Input: part model. Units: mm. Frame: model coordinates. A direction names the side the tool comes from. Round coordinates to 2 decimals unless told otherwise and drop trailing zeros. Loops run counter-clockwise (first coordinate to the right, second up) from the corner with the lowest first, then second, coordinate; pieces in that order, holes last. Notation, with made-up numbers: (30, 0) -> (77, 0) arc R7 cw to (77, 11) -> close; hole circle Ø7 at (55, 5). An arc over 180 degrees is marked (long way). One line per question, with ' | ' between items. Start each with the question number.
Q1. Access query for faces 1 (the face through (-47, -47, 0)), 2 (the face through (47, -47, 0.414)), 3 (the face through (-14.33, 109.11, 1.2)). Directions: +Z, -Z, +X, -X, +Y, -Y. A direction counts if a zero-diameter tool reaches every point of the face in a straight line with its end or side. Return the directions, or none.
Q2. Material intervals for L1, parallel to Y at x = 0, z = 1.15; L2, parallel to Z at x = 50, y = -100; L3, parallel to X at y = 99.5, z = 1.2, sorted ascending.
Q3. Contact query for a flat-ended pin moving along its axis: P1, Ø5, axis at x = 75.5, y = 37.5, coming from the +Z side. Output: stop coordinate, or through.
Q4. Cut plane A-A on y = 0. Return loops of the section in (x, z), and give its area (3 significant figures).
from build123d import *

# Parameters (mm, degrees)
F2_R     = 59.33948
F3_DEPTH = 25.4


with BuildPart() as f1:
    # F0 (on Front) → F1 (revolve)
    with BuildSketch(Plane.XZ):
        with BuildLine():
            Line((0, 0.414), (0, 0))
            Line((0, 0), (109.538073, 0))
            ThreePointArc((109.538073, 0), (109.89867, 0.149364), (110.048034, 0.509961))
            Line((110.048034, 0.509961), (110.048034, 1.878083))
            ThreePointArc((110.048034, 1.878083), (110.08374, 1.964284), (110.16994, 1.999989))
            Line((110.16994, 1.999989), (110.827769, 1.999989))
            Line((110.827769, 1.999989), (115.048034, 1.999989))
            Line((115.048034, 1.999989), (115.048034, 2.413989))
            Line((115.048034, 2.413989), (110.169929, 2.413989))
            ThreePointArc((110.169929, 2.413989), (109.790994, 2.257029), (109.634034, 1.878094))
            Line((109.634034, 1.878094), (109.634034, 0.509955))
            ThreePointArc((109.634034, 0.509955), (109.60593, 0.442105), (109.538079, 0.414))
            Line((109.538079, 0.414), (0, 0.414))
        make_face()
    revolve(axis=Axis((0, 0, 0.207), (0, 0, 1)))

    # F2 (on face) → F3 (cut)
    with BuildSketch(Plane.XY.offset(0.414)):
        Circle(F2_R)
    extrude(amount=-F3_DEPTH, mode=Mode.SUBTRACT)


solid = f1.part
Results:
1) face 1: -Z, +X, -X, +Y, -Y | face 2: +Z | face 3: -Z
2) L1: -110.05 to -109.63, 109.63 to 110.05 | L2: 2 to 2.41 | L3: -47.01 to -46.04, 46.04 to 47.01
3) P1: z = 0.41
4) outline: (-115.05, 2) -> (-110.17, 2) arc R0.12 cw to (-110.05, 1.88) -> (-110.05, 0.51) arc R0.51 ccw to (-109.54, 0) -> (-59.34, 0) -> (-59.34, 0.41) -> (-109.54, 0.41) arc R0.1 cw to (-109.63, 0.51) -> (-109.63, 1.88) arc R0.54 ccw to (-110.17, 2.41) -> (-115.05, 2.41) -> close; (59.34, 0) -> (109.54, 0) arc R0.51 ccw to (110.05, 0.51) -> (110.05, 1.88) arc R0.12 cw to (110.17, 2) -> (115.05, 2) -> (115.05, 2.41) -> (110.17, 2.41) arc R0.54 ccw to (109.63, 1.88) -> (109.63, 0.51) arc R0.1 cw to (109.54, 0.41) -> (59.34, 0.41) -> close | area: 47.6 mm^2
